Autodesk Inventor part; units mm, degrees
ref_plane "YZ Plane" through (0, 0, 0) normal (1, 0, 0) x (0, 1, 0)
ref_plane "XZ Plane" through (0, 0, 0) normal (0, 1, 0) x (-1, 0, 0)
ref_plane "XY Plane" through (0, 0, 0) normal (0, 0, 1) x (1, 0, 0)
sketch "Sketch3" plane through (0, 0, 0) normal (0, 1, 0) x (-1, 0, 0)
  circle A0 centre (0, 0) radius 4
  circle A1 centre (0, 0) radius 3
  dimension "d4" = 8
  dimension "d6" = 6
extrude "Extrusion2" add sketch "Sketch3" along normal blind 60
fillet "Fillet1" radius 0.3 2 edges at (4, 0, 0) (3, 0, 0)
fillet "Fillet2" radius 0.3 1 edges at (4, 60, 0)
fillet "Fillet3" radius 0.3 1 edges at (3, 60, 0)
properties part number "tube" material "Glass"
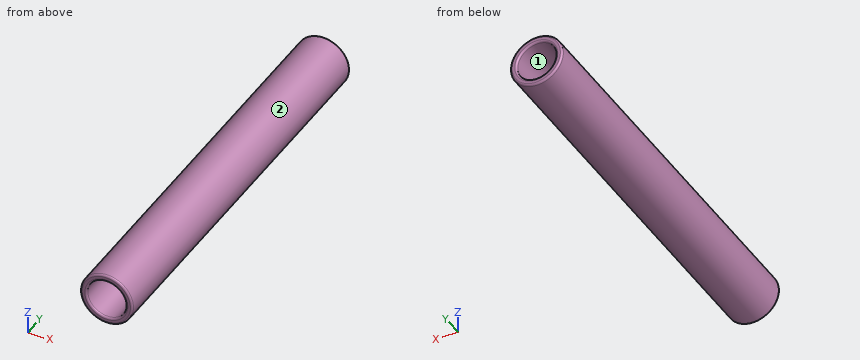
The listing builds one solid part. Answer for the finished solid, in the listing's coordinates (mm). Face numbers are marked on the shaded views. Give positions to 0.01 mm unless a question says otherwise; leave off trailing zeros. Order: outer loops, then holes, each group sorted by start corner. A loop starts at its lowest first (then second) coordinate and runs counter-clockwise, first axis right, second up. Notation, with made-up numbers: M 76.25,-21 L 110.25,-21 A25 cw 110.25,-5 Z; hole C 47.25,5.25 d5. An arc over 180 degrees is marked long. Put each result on its own line as item: value. Start each with the question number.
Item 1: For a pull along Z with two mould halves and no side action, classify the marked faces 1 and 2 as +Z half, -Z half, draft (parallel to the pull), parting line (faces both ways), or undercut.
Item 2: Find the intervals of material crossed by line 1 along X through (y, z) = (18, -0.25); line 2 along Z through (x, y) = (0, 39.5); line 3 along Y through (x, z) = (-0.25, 3.75), in increasing order.
Item 3: The part is cut by section A-A, the plane z = 0. Determine the outline of the cut face in (x, y).
Item 4: The part is cut by section B-B, the plane x = 0. Determine the outline of the cut face in (y, z), and give its area (3 significant figures).
Item 5: The part is cut by section C-C, the plane y = 56. Determine the outline of the cut face in (x, z).
Item 6: Flat-ended cylindrical pins translate along their axes: P1, Ø1.5, axis at y = 40, z = -1, coming from the +X side; P2, Ø3, axis at x = -2.5, y = 41, coming from the +Z side. Find the tip coordinate at first contact, or state that the pin passes through.
Answer key:
1. face 1: undercut
1. face 2: parting line
2. line 1: x = -3.99 to -2.99, 2.99 to 3.99
2. line 2: z = -4 to -3, 3 to 4
2. line 3: y = 0.01 to 59.99
3. outline: M -4,0.3 A0.3 ccw -3.7,0 L -3.3,0 A0.3 ccw -3,0.3 L -3,59.7 A0.3 ccw -3.3,60 L -3.7,60 A0.3 ccw -4,59.7 Z; M 3,0.3 A0.3 ccw 3.3,0 L 3.7,0 A0.3 ccw 4,0.3 L 4,59.7 A0.3 ccw 3.7,60 L 3.3,60 A0.3 ccw 3,59.7 Z
4. outline: M 0,-3.7 A0.3 ccw 0.3,-4 L 59.7,-4 A0.3 ccw 60,-3.7 L 60,-3.3 A0.3 ccw 59.7,-3 L 0.3,-3 A0.3 ccw 0,-3.3 Z; M 0,3.3 A0.3 ccw 0.3,3 L 59.7,3 A0.3 ccw 60,3.3 L 60,3.7 A0.3 ccw 59.7,4 L 0.3,4 A0.3 ccw 0,3.7 Z
4. area: 120 mm²
5. outline: C 0,0 d8; hole C 0,0 d6
6. P1: stops at x = 3.99
6. P2: stops at z = 3.87
